Check sheet for the modelled part. Datum: model origin and axes. Units: mm. A direction names the side the tool comes from. Round coordinates to 2 decimals unless told otherwise and drop trailing zeros. Write each loop counter-clockwise with the first axis right and the second up, starting at its lowest first coordinate (ties: lowest second). Pieces come first, ordered by that corner, then holes. Notation, with made-up numbers: M 69.25,13.25 L 111.25,13.25 A11 ccw 111.25,30.25 Z; hole C 52,9.25 d6. An arc over 180 degrees is marked long. One line per item, written item: value.
from build123d import *

# Parameters (mm, degrees)
SKETCH_1_W      = 41
SKETCH_1_H      = 40
SKETCH_1_W_2    = 33
SKETCH_1_H_2    = 32
EXTRUDE_5_DEPTH = 7
SKETCH_1_7_W    = 33
SKETCH_1_7_H    = 32
SKETCH_1_7_W_2  = 27
SKETCH_1_7_H_2  = 26
EXTRUDE_6_DEPTH = 3
SKETCH_1_9_R    = 1.75
EXTRUDE_7_DEPTH = 3


with BuildPart() as part:
    # 草图1 → 凸台-拉伸5 (new body)
    with BuildSketch(Plane.XY):
        with Locations((16.5, 16)):
            Rectangle(SKETCH_1_W, SKETCH_1_H)
        with Locations((16.5, 16)):
            Rectangle(SKETCH_1_W_2, SKETCH_1_H_2, mode=Mode.SUBTRACT)
    extrude(amount=EXTRUDE_5_DEPTH)

    # 草图1<7> → 凸台-拉伸6 (add)
    with BuildSketch(Plane.XY):
        with Locations((16.5, 16)):
            Rectangle(SKETCH_1_7_W, SKETCH_1_7_H)
        with Locations((16.5, 16)):
            Rectangle(SKETCH_1_7_W_2, SKETCH_1_7_H_2, mode=Mode.SUBTRACT)
    extrude(amount=EXTRUDE_6_DEPTH)

    # 草图1<9> → 凸台-拉伸7 (add)
    # profile 1 of 2: a face of its own
    with BuildSketch(Plane.XY):
        with BuildLine():
            Line((37, -4), (-4, -4))
            ThreePointArc((-4, -4), (16.5, -24.5), (37, -4))
        make_face()
        with Locations((16.5, -18)):
            Circle(SKETCH_1_9_R, mode=Mode.SUBTRACT)
        with Locations((16.5, -9)):
            Circle(SKETCH_1_9_R, mode=Mode.SUBTRACT)
    # profile 2 of 2: a face of its own
    with BuildSketch(Plane.XY):
        with BuildLine():
            ThreePointArc((37, 36), (16.5, 56.5), (-4, 36))
            Line((-4, 36), (37, 36))
        make_face()
        with Locations((16.5, 41)):
            Circle(SKETCH_1_9_R, mode=Mode.SUBTRACT)
        with Locations((16.5, 50)):
            Circle(SKETCH_1_9_R, mode=Mode.SUBTRACT)
    extrude(amount=EXTRUDE_7_DEPTH)


solid = part.part
Q1. Sectioned sample at A-A on y = 24.5. Enter the section's corners in (x, z).
Completed:
outline: M -4,0 L 3,0 L 3,3 L 0,3 L 0,7 L -4,7 Z; M 30,0 L 37,0 L 37,7 L 33,7 L 33,3 L 30,3 Z
Q2. Sectioned sample at C-C on z = 4.75. Enter the section's corners in (x, y), and give its area (3 significant figures).
Completed:
outline: M -4,-4 L 37,-4 L 37,36 L -4,36 Z; hole M 0,0 L 33,0 L 33,32 L 0,32 Z
area: 584 mm^2
Q3. Sectioned sample at B-B on x = 16.5. State how many separate pieces and enclosed holes the cut face has, and give its area (3 significant figures).
Completed:
separate pieces: 6
enclosed holes: 0
area: 155 mm^2
Q4. Draft check along X on faces 1 (the flat face through (37, 16, 3)), 2 (the flat face through (16, -1, 7)), 3 (the cylindrical face through (16.12, 39.29, 1.48)), 4 (the cylindrical face through (16.951, 56.495, 1.479)). Enter one of: pulls with the +X half, pulls with the -X half, needs draft (parallel to the pull), parting line crosses it, or undercut.
Completed:
face 1: pulls with the +X half
face 2: needs draft
face 3: undercut
face 4: parting line crosses it
Q5. Sectioned sample at D-D on x = 6.5. Enter the section's corners in (y, z), and give its area (3 significant figures).
Completed:
outline: M -21.9,0 L 3,0 L 3,3 L 0,3 L 0,7 L -4,7 L -4,3 L -21.9,3 Z; M 29,0 L 53.9,0 L 53.9,3 L 36,3 L 36,7 L 32,7 L 32,3 L 29,3 Z
area: 181 mm^2
Q6. Depth check by flat-ended pin: P1, Ø1.5, axis at x = 18.5, z = 2, coming from the -Y side; P2, Ø2, axis at x = 16.5, y = 41, coming from the +Z side; P3, Ø1.5, axis at x = 11, z = 1.5, coming from the +Y side; P4, Ø1.5, axis at x = 16.5, z = 4.5, coming from the -Y side. Enter the tip coordinate at first touch or a pass-through.
Completed:
P1: y = -24.46
P2: through
P3: y = 55.94
P4: y = -4
Q7. Access from +Z, -Z, +X, -X, +Y, -Y to the whole of each face (thin tool, end or side, straight path). Record for faces 5 (the flat face through (16, 29, 1)), 6 (the flat face through (16, 44, 3)), 7 (the flat face through (16, 0, 5)).
Completed:
face 5: +Z, -Z
face 6: +Z, +X, -X, +Y
face 7: +Z
Q8. Scan lines: line 1 (Y direction, x = 16.5, z = 2.05); line 2 (Y direction, x = 1.5, z = 6.5); line 3 (X direction, y = 20, z = 1.5). Record each from-to range of solid material in increasing order. Write a range as [from, to].
Completed:
line 1: [-24.5, -19.75], [-16.25, -10.75], [-7.25, 3], [29, 39.25], [42.75, 48.25], [51.75, 56.5]
line 2: [-4, 0], [32, 36]
line 3: [-4, 3], [30, 37]
